```python
from build123d import *
from build123d import SkipClean  # not in build123d's __all__

# Parameters (mm, degrees)
F0_W           = 116.3828
F0_H           = 76.2
F1_DEPTH       = 16.51
F2_R           = 12.7
F3_DEPTH       = 58.1914
F4_R           = 12.7
F6_DEPTH       = 15.875
F7_R           = 6.985
F10_DEPTH      = 53.34
F10_DEPTH_BACK = 53.34
F11_W          = 19.05
F11_H          = 5.715
F12_DEPTH      = 17.78
F13_W          = 20.32
F13_H          = 11.43
F14_DEPTH      = 1.27
F16_DEPTH      = 25.4
F17_R          = 5.08
F18_W          = 7.9625188272
F18_H          = 24.355364847
F18_W_2        = 74.197281152
F18_H_2        = 2.5465525687
F19_DEPTH      = 5.08
F20_T1_DEPTH   = 73.025
F20_T3_DEPTH   = 90.9828
F20_T6_ANGLE   = 90
F20_T8_ANGLE   = 90
F21_R          = 5.08
F22_R          = 13.97
F23_DEPTH      = 2.54
F24_R          = 13.97
F25_DEPTH      = 2.54
F26_R          = 9.525
F27_DEPTH      = 63.5
F29_DEPTH      = 25.4
F31_DEPTH      = 63.5


# Not quite as in the source:
# - a fillet or chamfer that OpenCascade refuses, or shapes differently, is made with other operations: its cross-section is extruded or revolved along the edge and cut away or added


with BuildPart() as f1:
    # F0 (on Top) → F1 (new body)
    with BuildSketch(Plane.XY):
        Rectangle(F0_W, F0_H)
    extrude(amount=F1_DEPTH)

    # F2 (on Right) → F3 (join, symmetric)
    with BuildSketch(Plane.YZ):
        with Locations((38.1, 0)):
            Circle(F2_R)
    extrude(amount=F3_DEPTH, both=True)

    # F4
    f4_edges = [f1.edges().sort_by_distance(p)[0] for p in [
        (-58.1914, -38.1, 8.255),
        (58.1914, -38.1, 8.255),
    ]]
    fillet(f4_edges, radius=F4_R)

    # F5 (on face) → F6 (cut)
    with BuildSketch(Plane(origin=(0, 0, 0), x_dir=(1, 0, 0), z_dir=(0, 0, -1))):
        with BuildLine():
            Line((-54.3814, 25.4), (-54.3814, -21.59))
            Line((-54.3814, -21.59), (54.3814, -21.59))
            Line((54.3814, -21.59), (54.3814, 25.4))
            ThreePointArc((54.3814, 25.4), (51.7775792847, 31.6861792847), (45.4914, 34.29))
            Line((45.4914, 34.29), (-45.4914, 34.29))
            ThreePointArc((-45.4914, 34.29), (-51.7775792847, 31.6861792847), (-54.3814, 25.4))
        make_face()
    extrude(amount=-F6_DEPTH, mode=Mode.SUBTRACT)

    # F8 (on Top) → F9 (revolve, cut)
    with BuildSketch(Plane.XY):
        Polygon((-30.48, 28.575), (-30.48, 25.4), (-30.48, 24.13), (30.48, 24.13), (30.48, 25.4), (30.48, 28.575), (24.13, 28.575), (19.05, 28.575), (19.05, 38.1), (0, 38.1), (-19.05, 38.1), (-19.05, 28.575), (-24.13, 28.575), align=None)
    revolve(axis=Axis((-9.525, 38.1, 0), (1, 0, 0)), mode=Mode.SUBTRACT)

    # F7 (on Right) → F10 (cut, two sides)
    with BuildSketch(Plane.YZ) as f10_sk:
        with Locations((38.1, 0)):
            Circle(F7_R)
    extrude(amount=F10_DEPTH, mode=Mode.SUBTRACT)
    extrude(f10_sk.sketch, amount=-F10_DEPTH_BACK, mode=Mode.SUBTRACT)

    # F11 (on face) → F12 (cut)
    with BuildSketch(Plane.XZ.offset(-21.59)):
        with Locations((44.8564, 4.1275)):
            Rectangle(F11_W, F11_H)
        with Locations((-44.8564, 4.1275)):
            Rectangle(F11_W, F11_H)
    extrude(amount=-F12_DEPTH, mode=Mode.SUBTRACT)

    # F13 (on face) → F14 (cut)
    with BuildSketch(Plane(origin=(54.3814, 0, 0), x_dir=(0, -1, 0), z_dir=(-1, 0, 0))):
        with Locations((-11.43, 10.16)):
            Rectangle(F13_W, F13_H)
    extrude(amount=-F14_DEPTH, mode=Mode.SUBTRACT)

    # F15 (on face) → F16 (cut)
    with BuildSketch(Plane(origin=(55.6514, 0, 0), x_dir=(0, -1, 0), z_dir=(-1, 0, 0))):
        Polygon((-17.145, 9.4234), (-5.715, 9.4234), (-5.715, 13.7922), (-11.43, 13.7922), (-17.145, 13.7922), align=None)
    extrude(amount=-F16_DEPTH, mode=Mode.SUBTRACT)

    # F17
    f17_edges = [f1.edges().sort_by_distance(p)[0] for p in [
        (-54.3814, -1.905, 15.875),
    ]]
    fillet(f17_edges, radius=F17_R)

    # F18 (on face) → F19 (join)
    with BuildSketch(Plane(origin=(0, 0, 15.875), x_dir=(1, 0, 0), z_dir=(0, 0, -1))):
        with Locations((52.2920594136, 10.7005844475)):
            Rectangle(F18_W, F18_H)
        Polygon((-35.9664, -19.1008), (-35.9664, -8.3696618676), (-39.6496931181, -8.3696618676), (-39.6496931181, -22.3802613997), (-21.43734819, -22.3802613997), (-21.43734819, -19.1008), align=None)
        with Locations((5.3238477558, 34.0265762843)):
            Rectangle(F18_W_2, F18_H_2)
    extrude(amount=F19_DEPTH)

    # F20: fillet of radius 3.81 on 1 edges, made by hand

    # F20_s2 → F20_t1 (cut)
    with BuildSketch(Plane.XZ.offset(-47.625)):
        with BuildLine():
            ThreePointArc((-58.1914, 12.7), (-57.0754768363, 15.3940768363), (-54.3814, 16.51))
            Line((-54.3814, 16.51), (-58.1914, 16.51))
            Line((-58.1914, 16.51), (-58.1914, 12.7))
        make_face()
        with BuildLine():
            ThreePointArc((58.1914, 12.7), (57.0754768363, 15.3940768363), (54.3814, 16.51))
            Line((54.3814, 16.51), (58.1914, 16.51))
            Line((58.1914, 16.51), (58.1914, 12.7))
        make_face()
    extrude(amount=F20_T1_DEPTH, mode=Mode.SUBTRACT)

    # F20_s4 → F20_t3 (cut)
    with BuildSketch(Plane.YZ.offset(-45.4914)):
        with BuildLine():
            ThreePointArc((-38.1, 12.7), (-36.9840768363, 15.3940768363), (-34.29, 16.51))
            Line((-34.29, 16.51), (-38.1, 16.51))
            Line((-38.1, 16.51), (-38.1, 12.7))
        make_face()
    extrude(amount=F20_T3_DEPTH, mode=Mode.SUBTRACT)

    # F20_s5 → F20_t6 (revolve, cut)
    with BuildSketch(Plane.XZ.offset(25.4)):
        with BuildLine():
            ThreePointArc((-58.1914, 12.7), (-57.0754768363, 15.3940768363), (-54.3814, 16.51))
            Line((-54.3814, 16.51), (-58.1914, 16.51))
            Line((-58.1914, 16.51), (-58.1914, 12.7))
        make_face()
    revolve(axis=Axis((-45.4914, -25.4, 16.51), (0, 0, 1)), revolution_arc=F20_T6_ANGLE, mode=Mode.SUBTRACT)

    # F20_s7 → F20_t8 (revolve, cut)
    with BuildSketch(Plane.XZ.offset(25.4)):
        with BuildLine():
            ThreePointArc((58.1914, 12.7), (57.0754768363, 15.3940768363), (54.3814, 16.51))
            Line((54.3814, 16.51), (58.1914, 16.51))
            Line((58.1914, 16.51), (58.1914, 12.7))
        make_face()
    revolve(axis=Axis((45.4914, -25.4, 16.51), (0, 0, -1)), revolution_arc=F20_T8_ANGLE, mode=Mode.SUBTRACT)

    # F21
    f21_edges = [f1.edges().sort_by_distance(p)[0] for p in [
        (58.1914, 47.080256, -8.980256),
        (-58.1914, 47.080256, -8.980256),
    ]]
    fillet(f21_edges, radius=F21_R)

    # F22 (on face) → F23 (cut)
    with BuildSketch(Plane(origin=(-58.1914, 0, 0), x_dir=(0, -1, 0), z_dir=(-1, 0, 0))):
        with Locations((-38.1, 0)):
            Circle(F22_R)
    extrude(amount=-F23_DEPTH, mode=Mode.SUBTRACT)

    # F24 (on face) → F25 (cut)
    with BuildSketch(Plane.YZ.offset(58.1914)):
        with Locations((38.1, 0)):
            Circle(F24_R)
    extrude(amount=-F25_DEPTH, mode=Mode.SUBTRACT)

    # F26 (on Right) → F27 (cut, symmetric)
    with BuildSketch(Plane.YZ):
        with Locations((38.1, 0)):
            Circle(F26_R)
    extrude(amount=F27_DEPTH, both=True, mode=Mode.SUBTRACT)

    # F28 (on face) → F29 (cut)
    with BuildSketch(Plane.XZ.offset(-21.59)):
        with BuildLine():
            ThreePointArc((12.065, 9.6555790053), (10.5771024484, 13.2476814537), (6.985, 14.7355790053))
            Line((6.985, 14.7355790053), (-6.985, 14.7355790053))
            ThreePointArc((-6.985, 14.7355790053), (-10.5771024484, 13.2476814537), (-12.065, 9.6555790053))
            Line((-12.065, 9.6555790053), (-12.065, 8.4972062227))
            ThreePointArc((-12.065, 8.4972062227), (-10.5771024484, 4.9051037742), (-6.985, 3.4172062227))
            Line((-6.985, 3.4172062227), (6.985, 3.4172062227))
            ThreePointArc((6.985, 3.4172062227), (10.5771024484, 4.9051037742), (12.065, 8.4972062227))
            Line((12.065, 8.4972062227), (12.065, 9.6555790053))
        make_face()
    extrude(amount=-F29_DEPTH, mode=Mode.SUBTRACT)

    # F30 (on Right) → F31 (cut, symmetric)
    with BuildSketch(Plane.YZ):
        with BuildLine():
            ThreePointArc((38.1, 12.446), (46.9006509986, -8.8006509986), (25.654, 0))
            Line((25.654, 0), (20.574, 0))
            Line((20.574, 0), (20.574, -20.574))
            Line((20.574, -20.574), (58.674, -20.574))
            Line((58.674, -20.574), (58.674, 17.526))
            Line((58.674, 17.526), (38.1, 17.526))
            Line((38.1, 17.526), (38.1, 12.446))
        make_face()
    with SkipClean():  # cleaning this boolean's faces spoils the solid; the shape is the same uncleaned
        extrude(amount=F31_DEPTH, both=True, mode=Mode.SUBTRACT)


solid = f1.part
```
Can you work these out from the model? Positions are in its coordinate system, mm. A direction names the side the tool comes from. Give positions to 0.01 mm unless a question says otherwise; leave off trailing zeros. Write each loop counter-clockwise with the first axis right and the second up, starting at its lowest first coordinate (ties: lowest second). Pieces come first, ordered by that corner, then holes. Notation, with made-up numbers: (19, 20) -> (60, 20) arc R21 ccw to (60, 55) -> close; hole circle Ø11 at (84.25, -28.5). An arc over 180 degrees is marked (long way). Write item = value, one per line.
(1) Thinking about a two-plate mould opening in Y: for faces 1 (the face through (1, 38.1, 15)), 2 (the face through (-58.191, 3, 6)), 3 (the face through (55.651, 12, 9)), which applies, released by +Y, released by -Y, zero draft, split by the parting line, or undercut?
Worked out:
face_1 = released by +Y
face_2 = zero draft
face_3 = undercut
(2) Suppose I cut it at C-C on x = 32. Write out the boundary of the cut face in (y, z) (3 decimals).
Worked out:
outline = (-38.1, 0) -> (-34.29, 0) -> (-34.29, 10.795) -> (-32.753, 10.795) -> (-32.753, 14.435) arc R5.08 cw to (-29.21, 15.875) -> (21.59, 15.875) -> (21.59, 0) -> (25.654, 0) arc R12.446 ccw (long way) to (38.1, 12.446) -> (38.1, 16.51) -> (-34.29, 16.51) arc R3.81 ccw to (-38.1, 12.7) -> close; hole circle Ø19.05 at (38.1, 0)
(3) For faces 4 (the face through (-0.637, -37.014, 15.364)), 5 (the face through (48.311, -11, 13)), 6 (the face through (0, 30, 14.736)), 7 (the face through (-45, 27, 6.985)), 8 (the face through (-55.651, 30, 6)), which set-ups out of +Z, -Z, +X, -X, +Y, -Y let a thin tool reach every point of the face, with its end or its side?
Worked out:
face_4 = +Z, +X, -X, -Y
face_5 = -Z
face_6 = +Y
face_7 = none
face_8 = -Z, -X, +Y
(4) I need wall thicknesses on probe 1 along Z at (x, y) = (36, 38); probe 2 along X at (y, z) = (40.5, -9.75); probe 3 along Z at (x, y) = (-44, 24) (3 decimals). Which ranges of each line are inside material? Lowest first, please. Write a range as from..to.
Worked out:
probe_1 = -12.45..-9.52, 9.52..16.51
probe_2 = -55.65..-30.48, 30.48..55.65
probe_3 = 0..1.27, 6.985..16.51
(5) Suppose I cut it at B-B on x = -16.5. Write out the boundary of the cut face in (y, z) (3 decimals).
Worked out:
outline = (-38.1, 0) -> (-34.29, 0) -> (-34.29, 10.795) -> (-32.753, 10.795) -> (-32.753, 14.435) arc R5.08 cw to (-29.21, 15.875) -> (21.59, 15.875) -> (21.59, 0) -> (24.13, 0) arc R13.97 cw to (38.1, 13.97) -> (38.1, 16.51) -> (-34.29, 16.51) arc R3.81 ccw to (-38.1, 12.7) -> close
(6) Suppose I cut it at D-D on z = -5.25. Count the separate pieces of the cut face and the enclosed holes in it, then the cut area to 3 significant figures.
Worked out:
separate_pieces = 4
enclosed_holes = 0
area = 335 mm^2
(7) I'm going to push flat-ended pins straight in: P1, Ø15, axis at y = 38.1, z = 0, coming from the +X side; P2, Ø1.8, axis at x = -38, z = 14.5, coming from the -Y side; P3, Ø8, axis at x = 53.5, y = -6, coming from the -Z side; P4, Ø4, axis at x = 21, z = 4, coming from the +Y side. Where does each tip first touch, or does it pass through?
Worked out:
P1 = through
P2 = -37.99
P3 = 0
P4 = 25.48
(8) Suppose I cut it at A-A on x = -1.5. Write out the boundary of the cut face in (y, z) (3 decimals).
Worked out:
outline = (-38.1, 0) -> (-34.29, 0) -> (-34.29, 10.795) -> (-32.753, 10.795) -> (-32.753, 14.435) arc R5.08 cw to (-29.21, 15.875) -> (21.59, 15.875) -> (21.59, 14.736) -> (38.1, 14.736) -> (38.1, 16.51) -> (-34.29, 16.51) arc R3.81 ccw to (-38.1, 12.7) -> close; (21.59, 0) -> (24.13, 0) arc R13.97 cw to (24.554, 3.417) -> (21.59, 3.417) -> close
